```python
from build123d import *

# Parameters (mm, degrees)
SKETCH1_R           = 2.5
SKETCH1_R_2         = 3.6
BOSS_EXTRUDE1_DEPTH = 3


with BuildPart() as part:
    # Sketch1 → Boss-Extrude1 (new body)
    with BuildSketch(Plane.XY):
        with BuildLine():
            Line((-60.14, -44), (60.14, -44))
            ThreePointArc((60.14, -44), (62.515878785, -43.015878785), (63.5, -40.64))
            Line((63.5, -40.64), (63.5, 40.64))
            ThreePointArc((63.5, 40.64), (62.515878785, 43.015878785), (60.14, 44))
            Line((60.14, 44), (-60.14, 44))
            ThreePointArc((-60.14, 44), (-62.515878785, 43.015878785), (-63.5, 40.64))
            Line((-63.5, 40.64), (-63.5, -40.64))
            ThreePointArc((-63.5, -40.64), (-62.515878785, -43.015878785), (-60.14, -44))
        make_face()
        Circle(SKETCH1_R, mode=Mode.SUBTRACT)
        with Locations((-49.845, 0)):
            Circle(SKETCH1_R, mode=Mode.SUBTRACT)
        with Locations((49.845, 0)):
            Circle(SKETCH1_R_2, mode=Mode.SUBTRACT)
        with Locations((-19.855, -30)):
            Circle(SKETCH1_R, mode=Mode.SUBTRACT)
        with Locations((19.855, -30)):
            Circle(SKETCH1_R_2, mode=Mode.SUBTRACT)
        with Locations((-29.85, -30)):
            Circle(SKETCH1_R, mode=Mode.SUBTRACT)
        with Locations((-39.85, -30)):
            Circle(SKETCH1_R, mode=Mode.SUBTRACT)
        with Locations((-49.845, -30)):
            Circle(SKETCH1_R, mode=Mode.SUBTRACT)
        with Locations((49.845, -30)):
            Circle(SKETCH1_R_2, mode=Mode.SUBTRACT)
        with Locations((39.85, -30)):
            Circle(SKETCH1_R_2, mode=Mode.SUBTRACT)
        with Locations((29.85, -30)):
            Circle(SKETCH1_R_2, mode=Mode.SUBTRACT)
        with Locations((49.845, 30)):
            Circle(SKETCH1_R_2, mode=Mode.SUBTRACT)
        with Locations((39.85, 30)):
            Circle(SKETCH1_R_2, mode=Mode.SUBTRACT)
        with Locations((29.85, 30)):
            Circle(SKETCH1_R_2, mode=Mode.SUBTRACT)
        with Locations((19.855, 30)):
            Circle(SKETCH1_R_2, mode=Mode.SUBTRACT)
        with Locations((-19.855, 30)):
            Circle(SKETCH1_R, mode=Mode.SUBTRACT)
        with Locations((-29.85, 30)):
            Circle(SKETCH1_R, mode=Mode.SUBTRACT)
        with Locations((-39.85, 30)):
            Circle(SKETCH1_R, mode=Mode.SUBTRACT)
        with Locations((-49.845, 30)):
            Circle(SKETCH1_R, mode=Mode.SUBTRACT)
        with Locations((-50.32, -20)):
            Circle(SKETCH1_R, mode=Mode.SUBTRACT)
        with Locations((-40.32, -20)):
            Circle(SKETCH1_R, mode=Mode.SUBTRACT)
        with Locations((-30.32, -20)):
            Circle(SKETCH1_R, mode=Mode.SUBTRACT)
        with Locations((-20.32, -20)):
            Circle(SKETCH1_R, mode=Mode.SUBTRACT)
        with Locations((50.32, -20)):
            Circle(SKETCH1_R, mode=Mode.SUBTRACT)
        with Locations((40.32, -20)):
            Circle(SKETCH1_R, mode=Mode.SUBTRACT)
        with Locations((30.32, -20)):
            Circle(SKETCH1_R, mode=Mode.SUBTRACT)
        with Locations((20.32, -20)):
            Circle(SKETCH1_R, mode=Mode.SUBTRACT)
        with Locations((50.32, 20)):
            Circle(SKETCH1_R, mode=Mode.SUBTRACT)
        with Locations((40.32, 20)):
            Circle(SKETCH1_R, mode=Mode.SUBTRACT)
        with Locations((30.32, 20)):
            Circle(SKETCH1_R, mode=Mode.SUBTRACT)
        with Locations((20.32, 20)):
            Circle(SKETCH1_R, mode=Mode.SUBTRACT)
        with Locations((-20.32, 20)):
            Circle(SKETCH1_R, mode=Mode.SUBTRACT)
        with Locations((-30.32, 20)):
            Circle(SKETCH1_R, mode=Mode.SUBTRACT)
        with Locations((-40.32, 20)):
            Circle(SKETCH1_R, mode=Mode.SUBTRACT)
        with Locations((-50.32, 20)):
            Circle(SKETCH1_R, mode=Mode.SUBTRACT)
        with Locations((-39.85, 0)):
            Circle(SKETCH1_R, mode=Mode.SUBTRACT)
        with Locations((-29.85, 0)):
            Circle(SKETCH1_R, mode=Mode.SUBTRACT)
        with Locations((-19.855, 0)):
            Circle(SKETCH1_R, mode=Mode.SUBTRACT)
        with Locations((39.85, 0)):
            Circle(SKETCH1_R_2, mode=Mode.SUBTRACT)
        with Locations((29.85, 0)):
            Circle(SKETCH1_R_2, mode=Mode.SUBTRACT)
        with Locations((19.855, 0)):
            Circle(SKETCH1_R_2, mode=Mode.SUBTRACT)
        with Locations((0, -20)):
            Circle(SKETCH1_R, mode=Mode.SUBTRACT)
        with Locations((0, 20)):
            Circle(SKETCH1_R, mode=Mode.SUBTRACT)
        with Locations((-10.16, -20)):
            Circle(SKETCH1_R, mode=Mode.SUBTRACT)
        with Locations((10.16, -20)):
            Circle(SKETCH1_R, mode=Mode.SUBTRACT)
        with Locations((10.16, 20)):
            Circle(SKETCH1_R, mode=Mode.SUBTRACT)
        with Locations((-10.16, 20)):
            Circle(SKETCH1_R, mode=Mode.SUBTRACT)
        with Locations((-10, 0)):
            Circle(SKETCH1_R, mode=Mode.SUBTRACT)
        with Locations((10, 0)):
            Circle(SKETCH1_R, mode=Mode.SUBTRACT)
        with Locations((0, -10)):
            Circle(SKETCH1_R, mode=Mode.SUBTRACT)
        with Locations((0, 10)):
            Circle(SKETCH1_R, mode=Mode.SUBTRACT)
        with Locations((-30.32, -10)):
            Circle(SKETCH1_R, mode=Mode.SUBTRACT)
        with Locations((-20.32, -10)):
            Circle(SKETCH1_R, mode=Mode.SUBTRACT)
        with Locations((30.32, -10)):
            Circle(SKETCH1_R, mode=Mode.SUBTRACT)
        with Locations((20.32, -10)):
            Circle(SKETCH1_R, mode=Mode.SUBTRACT)
        with Locations((30.32, 10)):
            Circle(SKETCH1_R, mode=Mode.SUBTRACT)
        with Locations((20.32, 10)):
            Circle(SKETCH1_R, mode=Mode.SUBTRACT)
        with Locations((-30.32, 10)):
            Circle(SKETCH1_R, mode=Mode.SUBTRACT)
        with Locations((-20.32, 10)):
            Circle(SKETCH1_R, mode=Mode.SUBTRACT)
        with Locations((-14.82, -14.82)):
            Circle(SKETCH1_R, mode=Mode.SUBTRACT)
        with Locations((14.82, -14.82)):
            Circle(SKETCH1_R, mode=Mode.SUBTRACT)
        with Locations((14.82, 14.82)):
            Circle(SKETCH1_R, mode=Mode.SUBTRACT)
        with Locations((-14.82, 14.82)):
            Circle(SKETCH1_R, mode=Mode.SUBTRACT)
        with BuildLine():
            Line((-10, -27.5), (10, -27.5))
            ThreePointArc((10, -27.5), (12.5, -30), (10, -32.5))
            Line((10, -32.5), (-10, -32.5))
            ThreePointArc((-10, -32.5), (-12.5, -30), (-10, -27.5))
        make_face(mode=Mode.SUBTRACT)
        with BuildLine():
            Line((-10, 27.5), (10, 27.5))
            ThreePointArc((10, 27.5), (12.5, 30), (10, 32.5))
            Line((10, 32.5), (-10, 32.5))
            ThreePointArc((-10, 32.5), (-12.5, 30), (-10, 27.5))
        make_face(mode=Mode.SUBTRACT)
        with BuildLine():
            Line((-3.25, -36.52), (3.25, -36.52))
            ThreePointArc((3.25, -36.52), (4.75, -38.02), (3.25, -39.52))
            Line((3.25, -39.52), (-3.25, -39.52))
            ThreePointArc((-3.25, -39.52), (-4.75, -38.02), (-3.25, -36.52))
        make_face(mode=Mode.SUBTRACT)
        with BuildLine():
            Line((-23.25, -36.52), (-16.75, -36.52))
            ThreePointArc((-16.75, -36.52), (-15.25, -38.02), (-16.75, -39.52))
            Line((-16.75, -39.52), (-23.25, -39.52))
            ThreePointArc((-23.25, -39.52), (-24.75, -38.02), (-23.25, -36.52))
        make_face(mode=Mode.SUBTRACT)
        with BuildLine():
            Line((23.25, -36.52), (16.75, -36.52))
            ThreePointArc((16.75, -36.52), (15.25, -38.02), (16.75, -39.52))
            Line((16.75, -39.52), (23.25, -39.52))
            ThreePointArc((23.25, -39.52), (24.75, -38.02), (23.25, -36.52))
        make_face(mode=Mode.SUBTRACT)
        with BuildLine():
            Line((-23.25, 36.52), (-16.75, 36.52))
            ThreePointArc((-16.75, 36.52), (-15.25, 38.02), (-16.75, 39.52))
            Line((-16.75, 39.52), (-23.25, 39.52))
            ThreePointArc((-23.25, 39.52), (-24.75, 38.02), (-23.25, 36.52))
        make_face(mode=Mode.SUBTRACT)
        with BuildLine():
            Line((-3.25, 36.52), (3.25, 36.52))
            ThreePointArc((3.25, 36.52), (4.75, 38.02), (3.25, 39.52))
            Line((3.25, 39.52), (-3.25, 39.52))
            ThreePointArc((-3.25, 39.52), (-4.75, 38.02), (-3.25, 36.52))
        make_face(mode=Mode.SUBTRACT)
        with BuildLine():
            Line((23.25, 36.52), (16.75, 36.52))
            ThreePointArc((16.75, 36.52), (15.25, 38.02), (16.75, 39.52))
            Line((16.75, 39.52), (23.25, 39.52))
            ThreePointArc((23.25, 39.52), (24.75, 38.02), (23.25, 36.52))
        make_face(mode=Mode.SUBTRACT)
    extrude(amount=BOSS_EXTRUDE1_DEPTH)


solid = part.part
```
Verification items for the finished model (mm, model axes). Round coordinates to 2 decimals unless told otherwise and drop trailing zeros. Write each loop counter-clockwise with the first axis right and the second up, starting at its lowest first coordinate (ties: lowest second). Pieces come first, ordered by that corner, then holes.
1. Section check B-B on y = 30. State how many separate pieces and enclosed holes the cut face has, plus the area to 3 significant figures.
2. Scan lines: L1, parallel to Y at x = 40.32, z = 1.05; L2, parallel to Y at x = 10.16, z = 1.85. Record each from-to range of solid material in increasing order.
3. Section check A-A on x = 50.5. Enter the section's corners in (y, z).
4. Draft check along Y on faces 1 (the cylindrical face through (62.49, -43.04, 1.48)), 2 (the cylindrical face through (-48.501, 32.108, 1.479)). Enter one of: +Y half, -Y half, draft (parallel to the pull), parting line (faces both ways), or undercut.
Answer:
1. separate pieces: 10
1. enclosed holes: 0
1. area: 160 mm2
2. L1: y = -44 to -33.57, -26.43 to -22.5, -17.5 to -3.57, 3.57 to 17.5, 22.5 to 26.43, 33.57 to 44
2. L2: y = -44 to -32.49, -27.51 to -22.5, -17.5 to -2.49, 2.49 to 17.5, 22.5 to 27.51, 32.49 to 44
3. outline: (-44, 0) - (-33.54, 0) - (-33.54, 3) - (-44, 3) - close; (-26.46, 0) - (-22.49, 0) - (-22.49, 3) - (-26.46, 3) - close; (-17.51, 0) - (-3.54, 0) - (-3.54, 3) - (-17.51, 3) - close; (3.54, 0) - (17.51, 0) - (17.51, 3) - (3.54, 3) - close; (22.49, 0) - (26.46, 0) - (26.46, 3) - (22.49, 3) - close; (33.54, 0) - (44, 0) - (44, 3) - (33.54, 3) - close
4. face 1: -Y half
4. face 2: undercut
